Source: three-view drawing plus pictorial views. Frame: mm from the lowest corner of the part. A direction names the side the tool comes from. Give positions to 0.01 mm unless a question says otherwise; leave off trailing zeros. Loops run counter-clockwise (first coordinate to the right, second up) from the corner with the lowest first, then second, coordinate; pieces in that order, holes last. Notation, with made-up numbers: M 0.5,29 L 23.5,29 A21 ccw 23.5,49 Z; hole C 10.5,10 d11. An arc over 180 degrees is marked long. Write item = value, one per line.
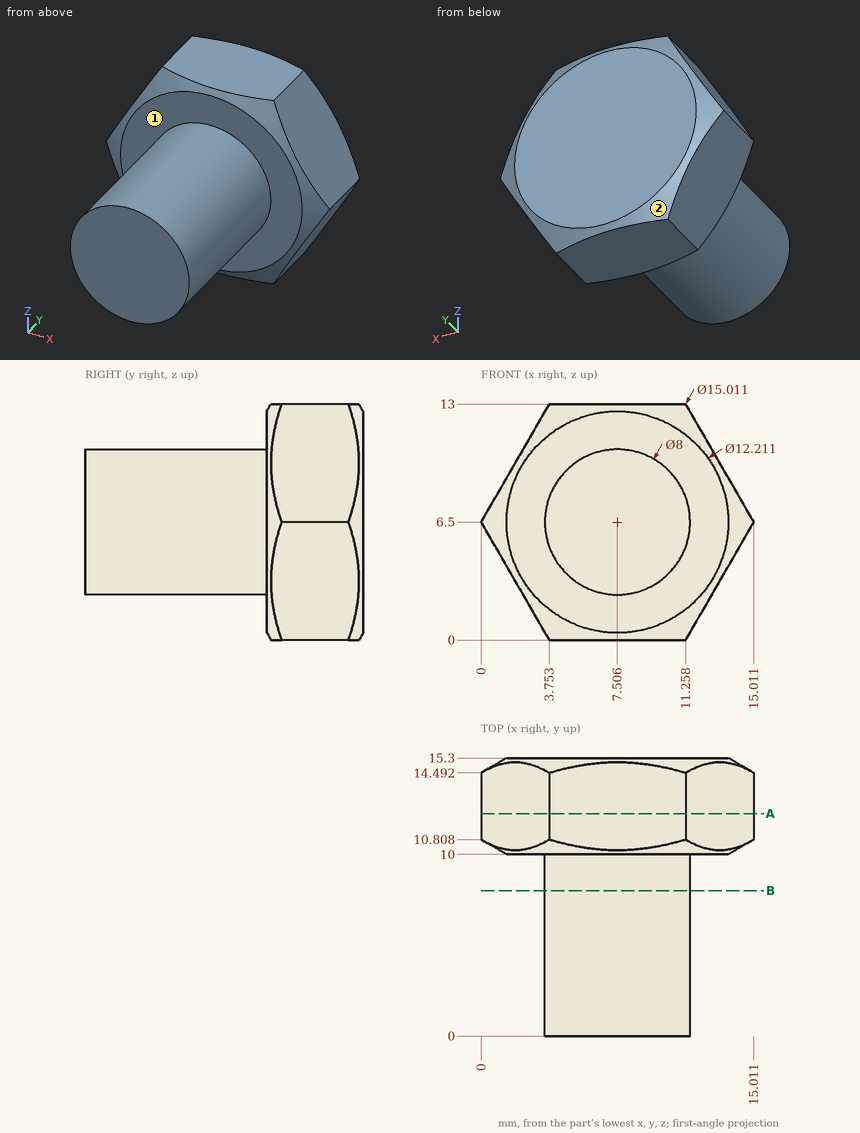
1. First-contact query: pin 1 Ø6 at (x, y) = (10, 1.5) entering from +Z; pin 2 Ø4 at (x, y) = (10.5, 3) entering from +Z (1 decimal); pin 3 Ø1 at (y, z) = (7, 5) entering from +X. Flat tips, straight axial feed; report the tip coordinate or a pass-through.
Derived:
pin_1 = 10.5
pin_2 = 10.4
pin_3 = 11.38
2. Reachability of the marked faces 1 and 2 from +Z, -Z, +X, -X, +Y, -Y: full face, straight path, thin tool, end or side. Return the list, or none.
Derived:
face_1 = -Y
face_2 = +Y
3. Material intervals for probe 1 along Y at (x, z) = (4.75, 10.25); probe 2 along X at (y, z) = (4, 6.5) (1 decimal); probe 3 along Y at (x, z) = (14, 7.5), sorted ascending. Write a range as from..to.
Derived:
probe_1 = 10..15.3
probe_2 = 3.5..11.5
probe_3 = 10.27..15.03
4. Cut plane A-A, the plane y = 12.25. Return the cut outline in (x, z).
Derived:
outline = M 0,6.5 L 3.75,0 L 11.26,0 L 15.01,6.5 L 11.26,13 L 3.75,13 Z
5. Cut plane B-B, the plane y = 8. Return the cut outline in (x, z) (1 decimal).
Derived:
outline = C 7.5,6.5 d8
